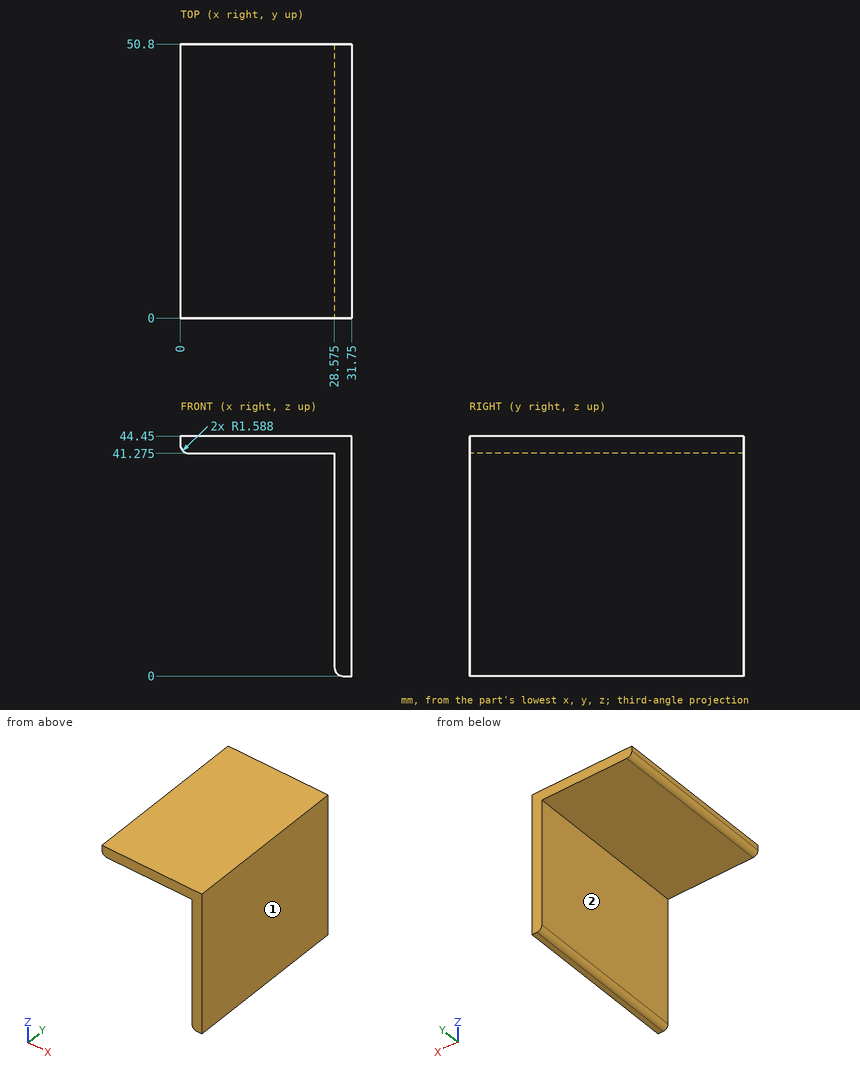
Job drawing, mm, ordinate dimensions from the low corner. One solid piece. A direction names the side the tool comes from. Round coordinates to 2 decimals unless told otherwise and drop trailing zeros. Answer in a Markdown table with one row per item.
1) Which spindle directions (+Z, -Z, +X, -X, +Y, -Y) get a long thin tool onto all of the face, cutting with end or side? Do the marked faces 1 and 2. Say none if no direction does.
Values:
| item | result |
|---|---|
| face 1 | +Z, -Z, +X, +Y, -Y |
| face 2 | -Z, -X, +Y, -Y |
2) Wall check: L1, parallel to Z at x = 30, y = 21. Give the ranges that are in metal, low to high.
Values:
| item | result |
|---|---|
| L1 | 0.01 to 44.45 |
3) Pin check, flat tips, straight feed: P1, Ø12, axis at y = 26.5, z = 17, coming from the -X side (1 decimal); P2, Ø13.5, axis at x = 8.5, y = 31, coming from the -Z side (1 decimal). Stop position of each tip, or through.
Values:
| item | result |
|---|---|
| P1 | x = 28.6 |
| P2 | z = 41.3 |
